Work out the finished part from the listing and answer in its coordinate system (mm). Face numbers are marked on the shaded views. Give positions to 0.01 mm unless a question says otherwise; leave off trailing zeros. Order: outer loops, then holes, each group sorted by start corner. A loop starts at its lowest first (then second) coordinate and runs counter-clockwise, first axis right, second up. Notation, with made-up numbers: (-9, -29.5) -> (-4, -29.5) arc R19 cw to (-4, -2.5) -> close; hole circle Ø4 at (63, -29.75). An arc over 180 degrees is marked (long way). Answer as CSV lines item,"result". Start each with the question number.
1. A cutting plane is placed at B-B (x = -29). Give the vertices of the cut face in (y, z), then the cut area to 3 significant figures.
2. For a pull along X with two mould halves and no side action, classify the marked faces 1 and 2 as released by +X, released by -X, zero draft, split by the parting line, or undercut.
3. A cutting plane is placed at A-A (x = 26.5). Give the vertices of the cut face in (y, z).
4. Flat-ended cylindrical pins translate along their axes: pin 1 (2.5 mm diameter, centred on x = -62, y = -10, fed in from -Z); pin 2 (0.8 mm diameter, centred on x = -61.5, z = -0.5, fed in from +Y); pin 3 (1.5 mm diameter, centred on x = 29, z = 2, fed in from -Y). Find the tip coordinate at first contact, or state that the pin passes through.
5. Find the intervals of material crossed by L1, parallel to X at y = -4.5, z = 1.9; L2, parallel to X at y = 12, z = -0.65; L3, parallel to X at y = -5.5, z = 1.6, in increasing order.
from build123d import *

# Parameters (mm, degrees)
SKETCH_R             = 1.000002
PAD_DEPTH            = 1.1
PAD001_DEPTH         = 3
SKETCH002_R          = 3.621622
SKETCH002_R_2        = 1.0871950633
SKETCH002_R_3        = 1.038663
SKETCH002_W          = 2.932263
SKETCH002_H          = 4.596517
SKETCH002_W_2        = 3.05114
SKETCH002_H_2        = 8.32128
SKETCH002_W_3        = 9.285799
SKETCH002_H_3        = 2.937828
SKETCH002_W_4        = 9.327248
SKETCH002_H_4        = 2.955594
PAD002_DEPTH         = 1
POCKET_DEPTH         = 2
PAD003_DEPTH         = 2
SKETCH005_W          = 3.065838
SKETCH005_H          = 10.665194
SKETCH005_W_2        = 6.121548
SKETCH005_H_2        = 3.191952
PAD004_DEPTH         = 1
BODY_PLACEMENT_ANGLE = 180


with BuildPart() as part:
    # Sketch → Pad (new body)
    with BuildSketch(Plane.XY):
        Polygon((-53.022964, 20.407351), (-52.9787547167, 0.2027583732), (-46.0602256559, -6.375196), (-46.0602256559, -18.4974481912), (63.976062776, -18.2566798895), (63.890903, 20.663168), align=None)
        with Locations((-44.255245, 18.462399)):
            Circle(SKETCH_R, mode=Mode.SUBTRACT)
        with Locations((61.870895, 18.823345)):
            Circle(SKETCH_R, mode=Mode.SUBTRACT)
        with Locations((62.086082, -16.283087)):
            Circle(SKETCH_R, mode=Mode.SUBTRACT)
        with Locations((25.123287, -16.858114)):
            Circle(SKETCH_R, mode=Mode.SUBTRACT)
        with Locations((-6.876536, -16.979681)):
            Circle(SKETCH_R, mode=Mode.SUBTRACT)
        with Locations((-44.183197, -16.667006)):
            Circle(SKETCH_R, mode=Mode.SUBTRACT)
        with Locations((-4.123168, 19.057377)):
            Circle(SKETCH_R, mode=Mode.SUBTRACT)
        with Locations((22.300682, 19.11718)):
            Circle(SKETCH_R, mode=Mode.SUBTRACT)
    extrude(amount=PAD_DEPTH)

    # Sketch001 → Pad001 (join)
    with BuildSketch(Plane.XY):
        Polygon((-36.844624, 16.276525), (-36.177216, 17.983372), (-35.306049, 18.757744), (-33.950901, 19.532116), (-10.728604, 19.532116), (-8.786971, 19.120708), (-7.915218, 18.248957), (-6.449088, 17.179077), (-5.181084, 16.941326), (-3.160203, 16.822451), (-1.297821, 17.377203), (0.401002, 18.814226), (1.471598, 19.5604), (2.704406, 19.884823), (17.074905, 19.884823), (18.534807, 19.564352), (19.313425, 18.915506), (20.319134, 18.104448), (21.519503, 16.871641), (22.849751, 15.56896), (23.460667, 14.53306), (23.726282, 13.072177), (25.027796, 13.072177), (25.027796, 18.169937), (25.208204, 19.013437), (25.662395, 19.564959), (26.246357, 19.889381), (54.529621, 19.889381), (54.947342, 19.840021), (55.269585, 19.637127), (57.763969, 17.23822), (58.038471, 16.641476), (58.06234, 16.247625), (58.06234, -10.412685), (57.961418, -11.086915), (57.531475, -11.428915), (56.710674, -11.888173), (26.824308, -11.888173), (25.868092, -11.772225), (25.310301, -11.081625), (25.097807, -10.364464), (23.955662, -10.444148), (23.955662, -13.832493), (23.614752, -14.78871), (23.056957, -15.851171), (21.835127, -16.913633), (19.616846, -17.367628), (16.833258, -17.367628), (4.714081, -17.367628), (-1.58584, -17.367628), (-2.892593, -16.866425), (-3.376577, -15.850059), (-3.376577, -14.122653), (-3.592077, -13.11694), (-4.143597, -12.532976), (-5.149311, -12.143668), (-32.677246, -12.143668), (-34.558903, -11.868008), (-35.661945, -10.894736), (-36.505447, -9.564599), (-36.844624, -8.440372), align=None)
    extrude(amount=PAD001_DEPTH)

    # Sketch002 (on Face5 of Pad001) → Pad002 (join)
    with BuildSketch(Plane.XY.offset(1.1)):
        with Locations((-41.301872, -7.651712)):
            Circle(SKETCH002_R)
        with Locations((61.760948, 11.435151)):
            Circle(SKETCH002_R_2)
        with Locations((61.793392, 4.39516)):
            Circle(SKETCH002_R_3)
        with Locations((61.727276, -2.725665)):
            Circle(SKETCH002_R_3)
        with Locations((61.740788, -9.574547)):
            Circle(SKETCH002_R_3)
        with Locations((-44.2495595, 11.9823365)):
            Rectangle(SKETCH002_W, SKETCH002_H)
        with Locations((-44.229748, 2.4723)):
            Rectangle(SKETCH002_W_2, SKETCH002_H_2)
        with Locations((-23.0629585, -16.513226)):
            Rectangle(SKETCH002_W_3, SKETCH002_H_3)
        with Locations((41.056557, -16.344444)):
            Rectangle(SKETCH002_W_4, SKETCH002_H_4)
    extrude(amount=PAD002_DEPTH)

    # Sketch003 (on Face107 of Pad002) → Pocket (cut)
    with BuildSketch(Plane.XY.offset(3)):
        Polygon((23.735168, 13.191908), (23.982185, -10.528876), (25.110214, -10.528876), (25.018686, 13.238607), align=None)
    extrude(amount=-POCKET_DEPTH, mode=Mode.SUBTRACT)

    # Sketch004 (on Face4 of Pocket) → Pad003 (join)
    with BuildSketch(Plane(origin=(0, 0, 0), x_dir=(1, 0, 0), z_dir=(0, 0, -1))):
        Polygon((-38.371834, 13.814776), (-39.017166, 13.360193), (-39.410694, 12.813627), (-39.520008, 12.4201), (-39.520008, -14.684528), (-38.980286, -15.923907), (-37.055988, -17.652515), (-36.142761, -18.174358), (-8.000727, -18.174358), (-7.087676, -17.71302), (-6.318431, -17.014458), (-6.318431, 12.349279), (-6.707822, 12.920823), (-7.176782, 13.433747), (-7.733671, 13.814776), align=None)
        Polygon((-5.504074, 12.586247), (-5.05245, 13.289701), (-4.55126, 13.737192), (30.83049, 13.737192), (31.573822, 13.584511), (32.339016, 12.666278), (32.701897, -14.178478), (32.288383, -15.067693), (31.512323, -15.647282), (-2.137218, -15.647282), (-5.504074, -13.009031), align=None)
        Polygon((33.824478, -11.830342), (34.277905, -12.79659), (35.083393, -13.136684), (56.290169, -13.136684), (57.16468, -12.83504), (57.492619, -12.026119), (57.492619, 11.701175), (56.447365, 12.796005), (35.343506, 12.796005), (34.37656, 12.325871), (33.824478, 11.411518), align=None)
    extrude(amount=PAD003_DEPTH)

    # Sketch005 (on Face4 of Pad003) → Pad004 (join)
    with BuildSketch(Plane(origin=(0, 0, 0), x_dir=(1, 0, 0), z_dir=(0, 0, -1))):
        with Locations((61.451113, -9.044624)):
            Rectangle(SKETCH005_W, SKETCH005_H)
        with Locations((52.262358, -16.842775)):
            Rectangle(SKETCH005_W_2, SKETCH005_H_2)
    extrude(amount=PAD004_DEPTH)


with BuildPart() as part_1:
    # Body placement: moved
    add(part.part.rotate(Axis((0, 0, 0), (0, 0, 1)), BODY_PLACEMENT_ANGLE))


solid = part_1.part
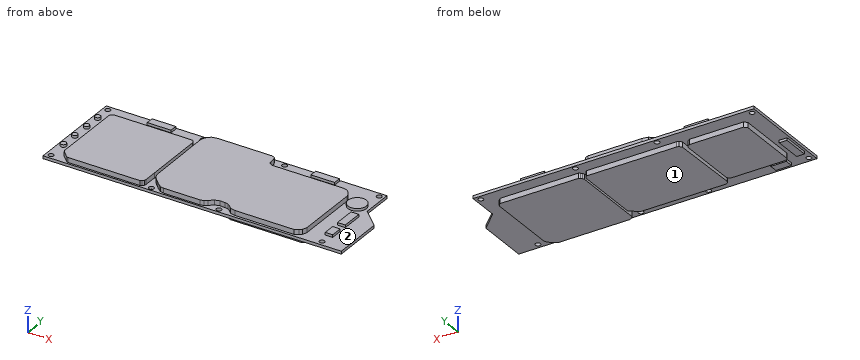
Answer sheet:
1,outline,"(-20.59, 0) -> (-15.65, 0) -> (-15.65, -2) -> (13.74, -2) -> (13.74, 0) -> (18.33, 0) -> (18.33, 1.1) -> (11.89, 1.1) -> (11.89, 3) -> (-19.89, 3) -> (-19.89, 1.1) -> (-20.59, 1.1) -> close"
1,area,"162 mm^2"
2,face 1,"zero draft"
2,face 2,"undercut"
3,outline,"(-20.47, 0) -> (-18.17, 0) -> (-18.17, -2) -> (13.81, -2) -> (13.81, 0) -> (18.45, 0) -> (18.45, 1.1) -> (17.98, 1.1) -> (17.98, 2.1) -> (15.04, 2.1) -> (15.04, 1.1) -> (12.14, 1.1) -> (12.14, 3) -> (-19.53, 3) -> (-19.53, 1.1) -> (-20.47, 1.1) -> close"
4,pin 1,"stops at z = -1"
4,pin 2,"stops at y = -3.71"
4,pin 3,"stops at y = -19.53"
5,L1,"x = -62.83 to -60.76, -58.06 to -25.05, -23.83 to 36.84, 42.7 to 45.76"
5,L2,"x = -57.21 to -34.18, -32.35 to 5.5, 6.32 to 39.52"
5,L3,"x = -58.06 to -25.05, -23.82 to 36.84, 42.7 to 45.76"
